from build123d import *

# Parameters (mm, degrees)
F0_R     = 13.3
F1_DEPTH = 4
F2_W     = 6
F2_H     = 4.4572373599
F3_DEPTH = 4.2
F4_R     = 2
F5_R     = 1.4
F6_DEPTH = 1.5


with BuildPart() as f1:
    # F0 (on Top) → F1 (new body)
    with BuildSketch(Plane.XY):
        Circle(F0_R)
        with BuildLine():
            Line((0, -8.5), (-8.5, -8.5))
            Line((-8.5, -8.5), (-8.5, -2.5))
            Line((-8.5, -2.5), (-10, -2.5))
            ThreePointArc((-10, -2.5), (-12.5, 0), (-10, 2.5))
            Line((-10, 2.5), (-8.5, 2.5))
            Line((-8.5, 2.5), (-8.5, 8.5))
            Line((-8.5, 8.5), (0, 8.5))
            Line((0, 8.5), (8.5, 8.5))
            Line((8.5, 8.5), (8.5, 2.5))
            Line((8.5, 2.5), (10, 2.5))
            ThreePointArc((10, 2.5), (11.767766953, 1.767766953), (12.5, 0))
            ThreePointArc((12.5, 0), (11.767766953, -1.767766953), (10, -2.5))
            Line((10, -2.5), (8.5, -2.5))
            Line((8.5, -2.5), (8.5, -8.5))
            Line((8.5, -8.5), (0, -8.5))
        make_face(mode=Mode.SUBTRACT)
    extrude(amount=F1_DEPTH)

    # F2 (on face) → F3 (join)
    with BuildSketch(Plane(origin=(0, 0, 0), x_dir=(1, 0, 0), z_dir=(0, 0, -1))):
        with Locations((0, 10.7286186799)):
            Rectangle(F2_W, F2_H)
    extrude(amount=F3_DEPTH)

    # F4
    f4_edges = [f1.edges().sort_by_distance(p)[0] for p in [
        (-3, -12.957237, -2.1),
        (-3, -8.5, -2.1),
        (3, -8.5, -2.1),
        (3, -12.957237, -2.1),
    ]]
    fillet(f4_edges, radius=F4_R)

    # F5 (on face) → F6 (join)
    with BuildSketch(Plane.XY.offset(4)):
        with BuildLine():
            ThreePointArc((0, 13.3), (9.4045201898, 9.4045201898), (13.3, 0))
            ThreePointArc((13.3, 0), (9.4045201898, -9.4045201898), (0, -13.3))
            Line((0, -13.3), (0, -13.75))
            Line((0, -13.75), (0, -17.4))
            Line((0, -17.4), (17.4, -17.4))
            Line((17.4, -17.4), (17.4, 17.4))
            Line((17.4, 17.4), (0, 17.4))
            Line((0, 17.4), (0, 13.3))
        make_face()
        with BuildLine():
            ThreePointArc((15.65, -13.75), (14.25, -15.15), (12.85, -13.75))
            ThreePointArc((12.85, -13.75), (14.25, -12.35), (15.65, -13.75))
        make_face(mode=Mode.SUBTRACT)
        with Locations((14.25, 13.75)):
            Circle(F5_R, mode=Mode.SUBTRACT)
        with BuildLine():
            Line((0, 8.5), (0, 13.3))
            ThreePointArc((0, 13.3), (-9.4045201898, 9.4045201898), (-13.3, 0))
            Line((-13.3, 0), (-12.5, 0))
            ThreePointArc((-12.5, 0), (-11.767766953, 1.767766953), (-10, 2.5))
            Line((-10, 2.5), (-8.5, 2.5))
            Line((-8.5, 2.5), (-8.5, 8.5))
            Line((-8.5, 8.5), (0, 8.5))
        make_face()
        with BuildLine():
            ThreePointArc((-13.3, 0), (-9.4045201898, 9.4045201898), (0, 13.3))
            Line((0, 13.3), (0, 17.4))
            Line((0, 17.4), (-17.4, 17.4))
            Line((-17.4, 17.4), (-17.4, -17.4))
            Line((-17.4, -17.4), (0, -17.4))
            Line((0, -17.4), (0, -13.75))
            Line((0, -13.75), (-12.85, -13.75))
            ThreePointArc((-12.85, -13.75), (-15.2399494937, -14.7399494937), (-14.25, -12.35))
            Line((-14.25, -12.35), (-14.25, 0))
            Line((-14.25, 0), (-13.3, 0))
        make_face()
        with BuildLine():
            ThreePointArc((-12.85, 13.75), (-13.2600505063, 12.7600505063), (-14.25, 12.35))
            ThreePointArc((-14.25, 12.35), (-15.2399494937, 14.7399494937), (-12.85, 13.75))
        make_face(mode=Mode.SUBTRACT)
        with BuildLine():
            Line((0, -13.75), (0, -13.3))
            ThreePointArc((0, -13.3), (-9.4045201898, -9.4045201898), (-13.3, 0))
            Line((-13.3, 0), (-14.25, 0))
            Line((-14.25, 0), (-14.25, -12.35))
            ThreePointArc((-14.25, -12.35), (-13.2600505063, -12.7600505063), (-12.85, -13.75))
            Line((-12.85, -13.75), (0, -13.75))
        make_face()
        with BuildLine():
            ThreePointArc((-13.3, 0), (-9.4045201898, -9.4045201898), (0, -13.3))
            Line((0, -13.3), (0, -8.5))
            Line((0, -8.5), (-8.5, -8.5))
            Line((-8.5, -8.5), (-8.5, -2.5))
            Line((-8.5, -2.5), (-10, -2.5))
            ThreePointArc((-10, -2.5), (-11.767766953, -1.767766953), (-12.5, 0))
            Line((-12.5, 0), (-13.3, 0))
        make_face()
    extrude(amount=-F6_DEPTH)


solid = f1.part
Verification items for the finished model (mm, model axes). A direction names the side the tool comes from. Coordinates: 2 decimals unless noted, no trailing zeros. Order: outer loops, then holes, each group sorted by start corner. A loop starts at its lowest first (then second) coordinate and runs counter-clockwise, first axis right, second up. Notation, with made-up numbers: M 20.5,85 L 29.5,85 A15 cw 29.5,89 Z; hole C 68.25,58 d9. An arc over 180 degrees is marked long. One line per item, written item: value. Start each with the question number.
Item 1: Sectioned sample at C-C (y = 5). Enter the section's corners in (x, z).
Item 2: Access from +Z, -Z, +X, -X, +Y, -Y to the whole of each face (thin tool, end or side, straight path). Record for faces 4 (the flat face through (0, -12.957, -2)), 5 (the cylindrical face through (2.43, -12.356, -2.129)), 6 (the cylindrical face through (12.286, -5.094, 1.232)), 7 (the cylindrical face through (-12.5, -0.1, 2)), 8 (the flat face through (0, 17.4, 3)).
Item 3: Mould release check, pull along X, two halves, no side actions. Record for faces 1 (the flat face through (9, -2.5, 2)), 2 (the flat face through (-17.4, 0, 3)), 3 (the flat face through (17.4, 0, 3)): released by +X, released by -X, zero draft, split by the parting line, or undercut.
Item 4: Sectioned sample at A-A (x = 14.25). Enter the section's corners in (y, z).
Item 5: Scan lines: probe 1 along Y at (x, z) = (-14.25, 3.5); probe 2 along Y at (x, z) = (1, 3); probe 3 along Z at (x, y) = (-15, -15). Record each from-to range of solid material in increasing order.
Item 6: Sectioned sample at B-B (z = 0.5). Enter the section's corners in (x, y), then the cut area to 3 significant figures.
Item 7: Sectioned sample at D-D (x = -10.5). Enter the section's corners in (y, z), then the cut area to 3 significant figures.
Item 8: Gauge pin test, flat ends, axial feed: pin 1 (1.5 mm diameter, centred on y = -12.5, z = 0.5, fed in from +X); pin 2 (1.5 mm diameter, centred on x = 5, z = -0.5, fed in from -Y); pin 3 (1.6 mm diameter, centred on x = -9.5, z = 1.5, fed in from -Y). Record the tip position at first contact, or that the pin passes through.
Conclusion:
1. outline: M -17.4,2.5 L -12.32,2.5 L -12.32,0 L -8.5,0 L -8.5,4 L -17.4,4 Z; M 8.5,0 L 12.32,0 L 12.32,2.5 L 17.4,2.5 L 17.4,4 L 8.5,4 Z
2. face 4: -Z, +X, -X, -Y
2. face 5: -Z, +X, -Y
2. face 6: -Z
2. face 7: +Z, -Z
2. face 8: +Z, -Z, +X, -X, +Y
3. face 1: undercut
3. face 2: released by -X
3. face 3: released by +X
4. outline: M -17.4,2.5 L -15.15,2.5 L -15.15,4 L -17.4,4 Z; M -12.35,2.5 L 12.35,2.5 L 12.35,4 L -12.35,4 Z; M 15.15,2.5 L 17.4,2.5 L 17.4,4 L 15.15,4 Z
5. probe 1: y = -17.4 to -15.15, -12.35 to 12.35, 15.15 to 17.4
5. probe 2: y = -17.4 to -8.5, 8.5 to 17.4
5. probe 3: z = 2.5 to 4
6. outline: C 0,0 d26.6; hole M -10,-2.5 L -8.5,-2.5 L -8.5,-8.5 L 8.5,-8.5 L 8.5,-2.5 L 10,-2.5 A2.5 ccw 10,2.5 L 8.5,2.5 L 8.5,8.5 L -8.5,8.5 L -8.5,2.5 L -10,2.5 A2.5 ccw Z
6. area: 232 mm^2
7. outline: M -17.4,2.5 L -8.16,2.5 L -8.16,0 L -2.45,0 L -2.45,4 L -17.4,4 Z; M 2.45,0 L 8.16,0 L 8.16,2.5 L 17.4,2.5 L 17.4,4 L 2.45,4 Z
7. area: 73.4 mm^2
8. pin 1: stops at x = 6.23
8. pin 2: stops at y = -12.54
8. pin 3: stops at y = -10.06
